The model under review builds one solid part; all positions refer to its coordinate system, in mm. Face numbers are marked on the shaded views. Round coordinates to 2 decimals unless told otherwise and drop trailing zeros. Order: outer loops, then holes, each group sorted by start corner. A loop starts at its lowest first (then second) coordinate and runs counter-clockwise, first axis right, second up. Notation, with made-up numbers: M 70.25,24 L 95.25,24 A18 cw 95.25,46 Z; hole C -27,84.25 d2. An arc over 180 degrees is marked long. Answer as a JSON object with one key per item and string values. Group by question number.
1. Clearance check with flat-ended pins moving along their axes: P1, Ø8.5, axis at x = -22.225, y = 0, coming from the -Z side (3 decimals); P2, Ø1.5, axis at y = -2.5, z = -0.5, coming from the -X side; P3, Ø3, axis at x = 25.4, y = -5.08, coming from the +Z side. State where each tip first meets the part, or that it passes through.
2. Add section B-B on z = 0. Give the number of separate pieces and of enclosed holes in the cut face, and give its area (3 significant figures).
3. To check wall thickness, follow probe 1 along Y at (x, z) = (25.4, 0.5) (1 decimal); probe 2 along Y at (x, z) = (-22.5, -0.5); probe 3 along Y at (x, z) = (26.5, -1.25) (3 decimals). State the ranges of each line that lie inside material, in increasing order. Write a range as [from, to].
4. Mouldability with a two-part tool opening along Y and no side actions: class the marked faces 1, 2 and 3 as released by +Y, released by -Y, zero draft, split by the parting line, or undercut.
5. Add section D-D on y = 2. State the section outline as (x, z) points (3 decimals).
6. Add section A-A on x = 25.4. State the section outline as (y, z) points (1 decimal), and give its area (3 significant figures).
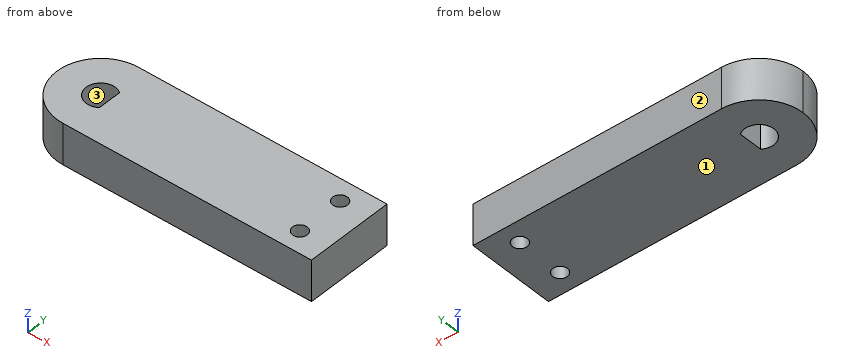
```python
from build123d import *

# Parameters (mm, degrees)
SKETCH1_W               = 63.5
SKETCH1_H               = 19.05
BOSS_EXTRUDE1_DEPTH     = 4.445
SKETCH2_R               = 1.5875
CUT_EXTRUDE1_DEPTH      = 12.7
FILLET1_R               = 9.525
CUT_EXTRUDE2_DEPTH      = 35.319385557
CUT_EXTRUDE2_DEPTH_BACK = 35.319385557


with BuildPart() as part:
    # Sketch1 → Boss-Extrude1 (new, symmetric)
    with BuildSketch(Plane.XY):
        Rectangle(SKETCH1_W, SKETCH1_H)
    extrude(amount=BOSS_EXTRUDE1_DEPTH, both=True)

    # Sketch2 → Cut-Extrude1 (cut)
    with BuildSketch(Plane.XY.offset(4.445)):
        with Locations((25.4, 5.08)):
            Circle(SKETCH2_R)
        with Locations((25.4, -5.08)):
            Circle(SKETCH2_R)
    extrude(amount=-CUT_EXTRUDE1_DEPTH, mode=Mode.SUBTRACT)

    # Fillet1
    fillet1_edges = [part.edges().sort_by_distance(p)[0] for p in [
        (-31.75, -9.525, 0),
        (-31.75, 9.525, 0),
    ]]
    fillet(fillet1_edges, radius=FILLET1_R - 0.0001)  # a hair under: the kernel refuses the full size

    # Sketch3 → Cut-Extrude2 (cut, two sides: drawn at the far end of the back side and taken through both)
    with BuildSketch(Plane.XY.offset(4.445).offset(-CUT_EXTRUDE2_DEPTH_BACK)):
        with BuildLine():
            Line((-20.32, 2.54), (-20.32, -2.54))
            ThreePointArc((-20.32, -2.54), (-25.4, 0), (-20.32, 2.54))
        make_face()
    extrude(amount=CUT_EXTRUDE2_DEPTH + CUT_EXTRUDE2_DEPTH_BACK, mode=Mode.SUBTRACT)


solid = part.part
```
Recorded:
{
 "1": {"P1": "stops at z = -4.445", "P2": "stops at x = -31.59", "P3": "passes through"},
 "2": {"separate pieces": "1", "enclosed holes": "3", "area": "1,130 mm²"},
 "3": {"probe 1": "y = [-9.5, -6.7], [-3.5, 3.5], [6.7, 9.5]", "probe 2": "y = [-9.52, -3.16], [3.16, 9.52]", "probe 3": "y = [-9.525, -6.225], [-3.935, 3.935], [6.225, 9.525]"},
 "4": {"face 1": "zero draft", "face 2": "released by +Y", "face 3": "undercut"},
 "5": {"outline": "M -31.538,-4.445 L -24.691,-4.445 L -24.691,4.445 L -31.538,4.445 Z; M -20.32,-4.445 L 31.75,-4.445 L 31.75,4.445 L -20.32,4.445 Z"},
 "6": {"outline": "M -9.5,-4.4 L -6.7,-4.4 L -6.7,4.4 L -9.5,4.4 Z; M -3.5,-4.4 L 3.5,-4.4 L 3.5,4.4 L -3.5,4.4 Z; M 6.7,-4.4 L 9.5,-4.4 L 9.5,4.4 L 6.7,4.4 Z", "area": "113 mm²"}
}
